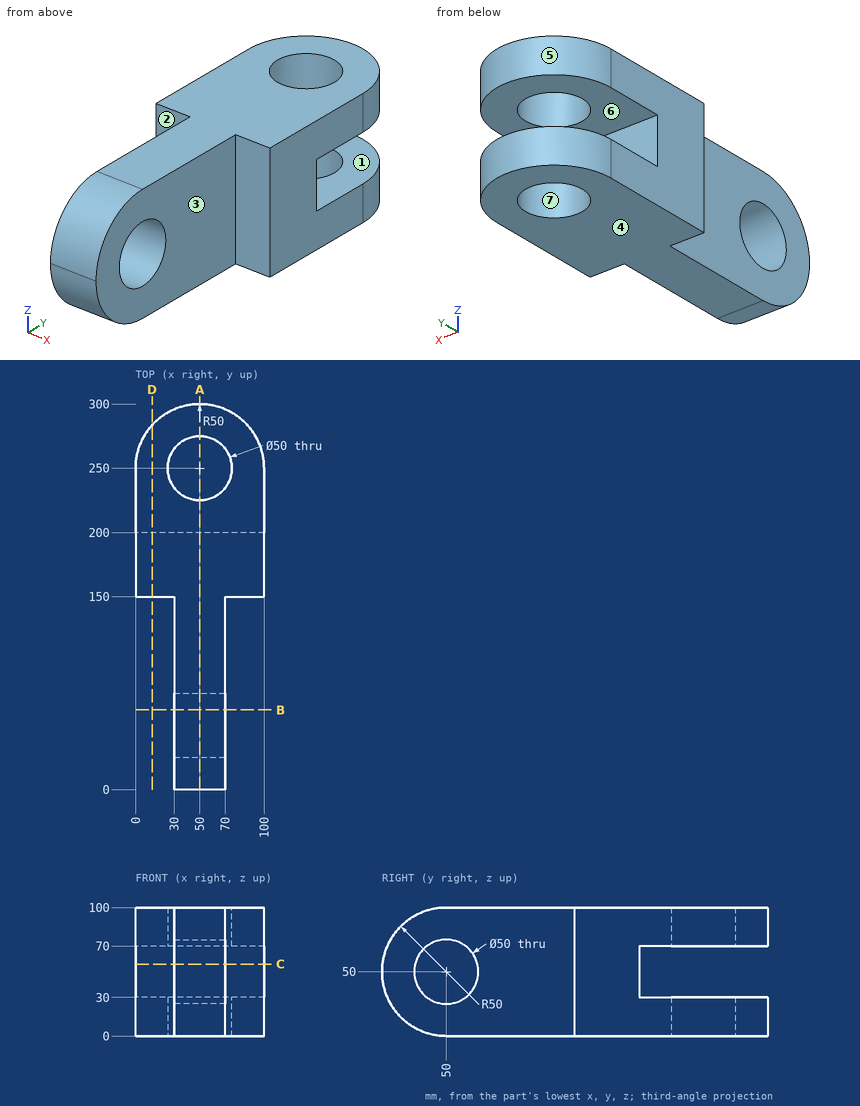
Check sheet for the drawn part. Datum: minimum x, y, z corner. Units: mm. A direction names the side the tool comes from. Give positions to 0.01 mm unless a question says otherwise; leave off trailing zeros. Order: outer loops, then holes, each group sorted by start corner. A loop starts at its lowest first (then second) coordinate and runs counter-clockwise, first axis right, second up.
1. Sectioned sample at B-B (y = 62). Record the boundary of the cut face in (x, z).
Completed:
outline: (30, 0) - (70, 0) - (70, 28.07) - (30, 28.07) - close; (30, 71.93) - (70, 71.93) - (70, 100) - (30, 100) - close
2. Access from +Z, -Z, +X, -X, +Y, -Y to the whole of each face (thin tool, end or side, straight path). Record for the marked faces 1, 2, 3 and 4.
Completed:
face 1: +X, -X, +Y
face 2: +Z, -Z, -X, -Y
face 3: +Z, -Z, +X, -Y
face 4: -Z, +X, -X, +Y, -Y
3. Scan lines: line 1 (X direction, y = 250, z = 84); line 2 (Z direction, x = 66.5, y = 288.5); line 3 (X direction, y = 42, z = 92). Record each from-to range of solid material in increasing order.
Completed:
line 1: x = 0 to 25, 75 to 100
line 2: z = 0 to 30, 70 to 100
line 3: x = 30 to 70
4. Draft check along Y on the marked faces 5, 6 and 7. Enter one of: pulls with the +Y half, pulls with the -Y half, needs draft (parallel to the pull), parting line crosses it, or undercut.
Completed:
face 5: pulls with the +Y half
face 6: needs draft
face 7: undercut
5. Depth check by flat-ended pin: pin 1 (5 mm diameter, centred on y = 268.5, z = 34, fed in from +X); pin 2 (4 mm diameter, centred on y = 108.5, z = 51.5, fed in from +X); pin 3 (15 mm diameter, centred on x = 91, z = 60, fed in from -Y); pin 4 (10 mm diameter, centred on x = 73.5, z = 31.5, fed in from +Y). Enter the tip coordinate at first touch or a pass-through.
Completed:
pin 1: passes through
pin 2: stops at x = 70
pin 3: stops at y = 150
pin 4: stops at y = 296.36
6. Sectioned sample at A-A (x = 50). Record the boundary of the cut face in (y, z), then the cut area to 3 significant figures.
Completed:
outline: (50, 0) - (225, 0) - (225, 30) - (200, 30) - (200, 70) - (225, 70) - (225, 100) - (50, 100) arc R50 ccw to start; (275, 0) - (300, 0) - (300, 30) - (275, 30) - close; (275, 70) - (300, 70) - (300, 100) - (275, 100) - close; hole circle Ø50 at (50, 50)
area: 20,000 mm2
7. Sectioned sample at C-C (z = 56). Record the boundary of the cut face in (x, y), then the cut area to 3 significant figures.
Completed:
outline: (0, 150) - (30, 150) - (30, 74.27) - (70, 74.27) - (70, 150) - (100, 150) - (100, 200) - (0, 200) - close; (30, 0.36) - (70, 0.36) - (70, 25.73) - (30, 25.73) - close
area: 9,040 mm2
8. Sectioned sample at D-D (x = 13). Record the boundary of the cut face in (y, z).
Completed:
outline: (150, 0) - (283.63, 0) - (283.63, 30) - (200, 30) - (200, 70) - (283.63, 70) - (283.63, 100) - (150, 100) - close
